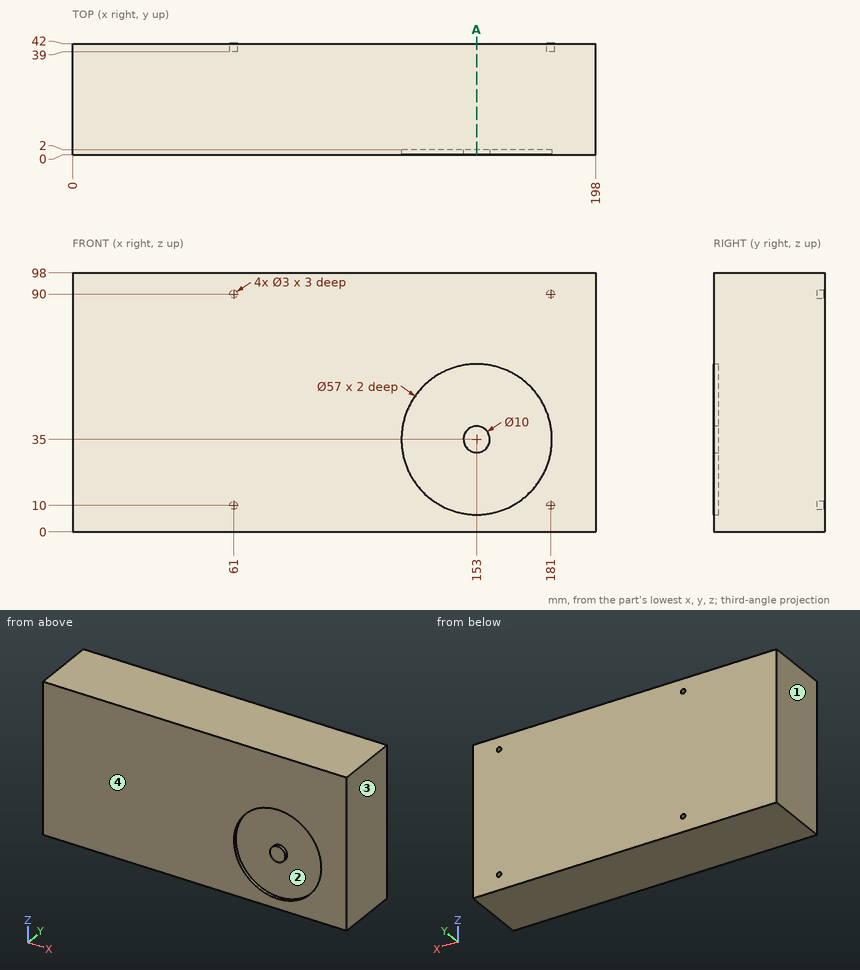
Input: dimensioned drawing with shaded views. Units: mm. Origin: part minimum x, y, z. Give positions to 0.01 mm unless a question says otherwise; leave off trailing zeros. Write each loop counter-clockwise with the first axis right and the second up, starting at its lowest first coordinate (ties: lowest second). Pieces come first, ordered by that corner, then holes.
Q1. Material intervals for probe 1 along X at (y, z) = (40.4, 10); probe 2 along Z at (x, y) = (181, 39.8); probe 3 along X at (y, z) = (1.5, 35), sorted ascending.
Q2. Pull-direction query (X, two-part tool) for the marked faces 1, 2, 3 and 4; classes: pulls with the +X half, pulls with the -X half, needs draft (parallel to the pull), parting line crosses it, or undercut.
Q3. First-contact query: P1, Ø1.5, axis at x = 61, z = 9.5, coming from the +Y side. Flat tip, straight axial feed; report the tip coordinate or a pass-through.
Q4. Section A-A, the plane x = 153. Output: boundary loops of the cut face in (y, z).
Filled in:
1. probe 1: x = 0 to 59.5, 62.5 to 179.5, 182.5 to 198
1. probe 2: z = 0 to 8.5, 11.5 to 88.5, 91.5 to 98
1. probe 3: x = 0 to 124.5, 148 to 158, 181.5 to 198
2. face 1: pulls with the -X half
2. face 2: undercut
2. face 3: pulls with the +X half
2. face 4: needs draft
3. P1: stops at y = 39
4. outline: (0, 0) - (42, 0) - (42, 98) - (0, 98) - (0, 63.5) - (2, 63.5) - (2, 40) - (0, 40) - (0, 30) - (2, 30) - (2, 6.5) - (0, 6.5) - close
